from build123d import *

# Parameters (mm, degrees)
SKETCH_1_W          = 42
SKETCH_1_H          = 38
EXTRUDE_1_DEPTH     = 3.5
EXTRUDE_2_DEPTH     = 4
SKETCH_3_W          = 35
SKETCH_3_H          = 31
CUT_EXTRUDE_1_DEPTH = 1.5
SKETCH_4_W          = 42
SKETCH_4_H          = 38
SKETCH_4_W_2        = 35
SKETCH_4_H_2        = 31
EXTRUDE_3_DEPTH     = 4
SKETCH_6_W          = 42
SKETCH_6_H          = 38
EXTRUDE_4_DEPTH     = 2
SKETCH_7_W          = 4
SKETCH_7_H          = 25
CUT_EXTRUDE_2_DEPTH = 3.5
SKETCH_8_W          = 3.5
SKETCH_8_H          = 2.331830178
CUT_EXTRUDE_3_DEPTH = 3.5
CUT_EXTRUDE_4_DEPTH = 10
SKETCH_10_W         = 1.5
SKETCH_10_H         = 31
EXTRUDE_5_DEPTH     = 5


with BuildPart() as part:
    # 草图1 → 凸台-拉伸1 (new body)
    with BuildSketch(Plane.XY):
        with Locations((21, 19)):
            Rectangle(SKETCH_1_W, SKETCH_1_H)
    extrude(amount=EXTRUDE_1_DEPTH)

    # 草图2 → 凸台-拉伸2 (add)
    with BuildSketch(Plane.XY.offset(3.5)):
        Polygon((0, 21), (0, 19), (0, 17), (3.5, 17), (3.5, 21), align=None)
        Polygon((42, 17), (42, 19), (42, 21), (38.5, 21), (38.5, 17), align=None)
    extrude(amount=EXTRUDE_2_DEPTH)

    # 草图3 → 切除-拉伸1 (cut)
    with BuildSketch(Plane.XY.offset(3.5)):
        with Locations((21, 19)):
            Rectangle(SKETCH_3_W, SKETCH_3_H)
    extrude(amount=-CUT_EXTRUDE_1_DEPTH, mode=Mode.SUBTRACT)

    # 草图4 → 凸台-拉伸3 (add)
    with BuildSketch(Plane(origin=(0, 0, 0), x_dir=(-1, 0, 0), z_dir=(0, 0, -1))):
        with Locations((-21, 19)):
            Rectangle(SKETCH_4_W, SKETCH_4_H)
        with Locations((-21, 19)):
            Rectangle(SKETCH_4_W_2, SKETCH_4_H_2, mode=Mode.SUBTRACT)
    extrude(amount=EXTRUDE_3_DEPTH)

    # 草图6 → 凸台-拉伸4 (add)
    with BuildSketch(Plane(origin=(0, 0, -4), x_dir=(-1, 0, 0), z_dir=(0, 0, -1))):
        with Locations((-21, 19)):
            Rectangle(SKETCH_6_W, SKETCH_6_H)
    extrude(amount=EXTRUDE_4_DEPTH)

    # 草图7 → 切除-拉伸2 (cut)
    with BuildSketch(Plane.ZY):
        with Locations((-2, 16)):
            Rectangle(SKETCH_7_W, SKETCH_7_H)
    extrude(amount=-CUT_EXTRUDE_2_DEPTH, mode=Mode.SUBTRACT)

    # 草图8 → 切除-拉伸3 (cut)
    with BuildSketch(Plane.ZY):
        with Locations((1.75, 4.665915089)):
            Rectangle(SKETCH_8_W, SKETCH_8_H)
    extrude(amount=-CUT_EXTRUDE_3_DEPTH, mode=Mode.SUBTRACT)

    # 草图9 → 切除-拉伸4 (cut)
    with BuildSketch(Plane(origin=(0, 0, -6), x_dir=(-1, 0, 0), z_dir=(0, 0, -1))):
        with BuildLine():
            Line((-38.044699478, 27), (-29.186779496, 27))
            ThreePointArc((-29.186779496, 27), (-28.186779496, 26), (-29.186779496, 25))
            Line((-29.186779496, 25), (-38.044699478, 25))
            ThreePointArc((-38.044699478, 25), (-39.044699478, 26), (-38.044699478, 27))
        make_face()
        with BuildLine():
            Line((-38.044699478, 30.5), (-29.186779496, 30.5))
            ThreePointArc((-29.186779496, 30.5), (-28.186779496, 29.5), (-29.186779496, 28.5))
            Line((-29.186779496, 28.5), (-38.044699478, 28.5))
            ThreePointArc((-38.044699478, 28.5), (-39.044699478, 29.5), (-38.044699478, 30.5))
        make_face()
        with BuildLine():
            Line((-38.044699478, 34), (-29.186779496, 34))
            ThreePointArc((-29.186779496, 34), (-28.186779496, 33), (-29.186779496, 32))
            Line((-29.186779496, 32), (-38.044699478, 32))
            ThreePointArc((-38.044699478, 32), (-39.044699478, 33), (-38.044699478, 34))
        make_face()
    extrude(amount=-CUT_EXTRUDE_4_DEPTH, mode=Mode.SUBTRACT)

    # 草图10 → 凸台-拉伸5 (add)
    with BuildSketch(Plane(origin=(0, 0, 0), x_dir=(-1, 0, 0), z_dir=(0, 0, -1))):
        with Locations((-27.23390418, 19)):
            Rectangle(SKETCH_10_W, SKETCH_10_H)
    extrude(amount=EXTRUDE_5_DEPTH)


solid = part.part
Read the model definition and answer for the solid it produces. Units are mm, in the model's axes. A direction names the side the tool comes from. Give positions to 0.01 mm unless a question says otherwise; leave off trailing zeros. Write each loop counter-clockwise with the first axis right and the second up, starting at its lowest first coordinate (ties: lowest second). Pieces come first, ordered by that corner, then holes. Notation, with made-up numbers: M 58.25,-15 L 110.25,-15 A30 ccw 110.25,23 Z; hole C 63.5,61 d9. An arc over 180 degrees is marked long. One line per item, written item: value. Start each with the question number.
(1) Flat-ended cylindrical pins translate along their axes: pin 1 Ø1.6 at (y, z) = (4.5, 0.5) entering from -X; pin 2 Ø2 at (x, y) = (27, 6) entering from +Z; pin 3 Ø2 at (y, z) = (19.5, -1.5) entering from -X. Find the tip coordinate at first contact, or state that the pin passes through.
(2) Find section C-C (x = 13.5). Determine the outline of the cut face in (y, z), plus the area to 4 significant figures.
(3) Find section A-A (y = 29.5). Determine the outline of the cut face in (x, z), plus the area to 3 significant figures.
(4) Find section B-B (z = -3.5). Determine the outline of the cut face in (x, y).
(5) Find the intervals of material crossed by line 1 (X direction, y = 14.5, z = -2); line 2 (Y direction, x = 34, z = 3); line 3 (Z direction, x = 7.5, y = 7.5), in increasing order.
(6) Determine the mould class of faces 5 (the flat face through (2, 17, 5)), 6 (the cylindrical face through (28.187, 33.022, -5.014)), 7 (the flat face through (21, 38, -1)), 8 (the flat face through (42, 19, -1)) for opening direction Y: pulls with the +Y half, pulls with the -Y half, needs draft (parallel to the pull), parting line crosses it, or undercut.
(7) A tool of negligible diameter and unlimited length cuts with its end or side. For faces 1 (the flat face through (34, 27, 1)), 2 (the flat face through (2, 5.832, 2)), 3 (the flat face through (2, 11, 3.5)), 4 (the flat face through (13, 19, -4)), from which of +Z, -Z, +X, -X, +Y, -Y can it reach the whole face along a straight path? Write none if from no direction.
(8) Find section D-D (z = 6). Determine the outline of the cut face in (x, y).
Results below:
1. pin 1: stops at x = 3.5
1. pin 2: stops at z = 2
1. pin 3: stops at x = 26.48
2. outline: M 0,-6 L 38,-6 L 38,3.5 L 34.5,3.5 L 34.5,2 L 3.5,2 L 3.5,3.5 L 0,3.5 Z; hole M 3.5,-4 L 34.5,-4 L 34.5,0 L 3.5,0 Z
2. area: 190.5 mm^2
3. outline: M 0,-6 L 28.19,-6 L 28.19,-4 L 27.98,-4 L 27.98,0 L 28.19,0 L 28.19,2 L 3.5,2 L 3.5,3.5 L 0,3.5 Z; M 39.04,-6 L 42,-6 L 42,3.5 L 39.04,3.5 Z; hole M 3.5,-4 L 26.48,-4 L 26.48,0 L 3.5,0 Z
3. area: 166 mm^2
4. outline: M 0,0 L 42,0 L 42,38 L 0,38 L 0,28.5 L 3.5,28.5 L 3.5,34.5 L 26.48,34.5 L 26.48,3.5 L 0,3.5 Z; hole M 27.98,3.5 L 38.5,3.5 L 38.5,25.11 A1 ccw 38.5,26.89 L 38.5,28.61 A1 ccw 38.5,30.39 L 38.5,32.11 A1 ccw 38.5,33.89 L 38.5,34.5 L 27.98,34.5 Z
5. line 1: x = 26.48 to 27.98, 38.5 to 42
5. line 2: y = 0 to 3.5, 34.5 to 38
5. line 3: z = -6 to -4, 0 to 2
6. face 5: pulls with the -Y half
6. face 6: undercut
6. face 7: pulls with the +Y half
6. face 8: needs draft
7. face 1: +Z, -Z
7. face 2: +Z, -X
7. face 3: +Z, +X, -X, -Y
7. face 4: none
8. outline: M 0,17 L 3.5,17 L 3.5,21 L 0,21 Z; M 38.5,17 L 42,17 L 42,21 L 38.5,21 Z
